from build123d import *

# Parameters (mm, degrees)
SKETCH1_R           = 150
SKETCH1_W           = 33
SKETCH1_H           = 33
BOSS_EXTRUDE1_DEPTH = 5
SKETCH4_R           = 1.5
CUT_EXTRUDE1_DEPTH  = 55
CIRPATTERN1_COUNT   = 12
CUT_EXTRUDE2_REACH  = 214.368
SKETCH5_W           = 20
SKETCH5_H           = 5
SKETCH5_W_2         = 5
SKETCH5_H_2         = 20
CUT_EXTRUDE3_DEPTH  = 10
BOSS_EXTRUDE2_DEPTH = 5
CUT_EXTRUDE4_DEPTH  = 5
BOSS_EXTRUDE3_DEPTH = 15
SKETCH11_W          = 22.5
SKETCH11_H          = 8
BOSS_EXTRUDE4_DEPTH = 3


with BuildPart() as part:
    # Sketch1 → Boss-Extrude1 (new, symmetric)
    with BuildSketch(Plane.XY):
        Circle(SKETCH1_R)
        Polygon((37.460580838, 97.883629292), (66.039419162, 81.383629292), (82.539419162, 109.962467617), (53.960580838, 126.462467617), align=None, mode=Mode.SUBTRACT)
        with Locations((0, 120)):
            Rectangle(SKETCH1_W, SKETCH1_H, mode=Mode.SUBTRACT)
        Polygon((81.383629292, 66.039419162), (97.883629292, 37.460580838), (126.462467617, 53.960580838), (109.962467617, 82.539419162), align=None, mode=Mode.SUBTRACT)
        with Locations((120, 0)):
            Rectangle(SKETCH1_W, SKETCH1_H, mode=Mode.SUBTRACT)
        Polygon((97.883629292, -37.460580838), (81.383629292, -66.039419162), (109.962467617, -82.539419162), (126.462467617, -53.960580838), align=None, mode=Mode.SUBTRACT)
        Polygon((66.039419162, -81.383629292), (37.460580838, -97.883629292), (53.960580838, -126.462467617), (82.539419162, -109.962467617), align=None, mode=Mode.SUBTRACT)
        with Locations((0, -120)):
            Rectangle(SKETCH1_W, SKETCH1_H, mode=Mode.SUBTRACT)
        Polygon((-37.460580838, -97.883629292), (-66.039419162, -81.383629292), (-82.539419162, -109.962467617), (-53.960580838, -126.462467617), align=None, mode=Mode.SUBTRACT)
        Polygon((-81.383629292, -66.039419162), (-97.883629292, -37.460580838), (-126.462467617, -53.960580838), (-109.962467617, -82.539419162), align=None, mode=Mode.SUBTRACT)
        with Locations((-120, 0)):
            Rectangle(SKETCH1_W, SKETCH1_H, mode=Mode.SUBTRACT)
        Polygon((-97.883629292, 37.460580838), (-81.383629292, 66.039419162), (-109.962467617, 82.539419162), (-126.462467617, 53.960580838), align=None, mode=Mode.SUBTRACT)
        Polygon((-66.039419162, 81.383629292), (-37.460580838, 97.883629292), (-53.960580838, 126.462467617), (-82.539419162, 109.962467617), align=None, mode=Mode.SUBTRACT)
    extrude(amount=BOSS_EXTRUDE1_DEPTH, both=True)

    # Sketch4 → Cut-Extrude1 (cut)
    with BuildSketch(Plane(origin=(0, -150, 0), x_dir=(-1, 0, 0), z_dir=(0, -1, 0))):
        with Locations(Location((0, 0, 0), (0, 0, 90))):
            Circle(SKETCH4_R)
    cut_extrude1 = extrude(amount=-CUT_EXTRUDE1_DEPTH, mode=Mode.SUBTRACT)

    # CirPattern1: Cut-Extrude1 ×12 about axis
    cirpattern1_axis = Axis((0, 0, 0), (0, 0, 1))
    for i in range(1, CIRPATTERN1_COUNT):
        add(cut_extrude1.rotate(cirpattern1_axis, i * 360 / CIRPATTERN1_COUNT), mode=Mode.SUBTRACT)

    # Sketch5 → Cut-Extrude2 (cut, up to next)
    with BuildSketch(Plane(origin=(0, 0, -5), x_dir=(-1, 0, 0), z_dir=(0, 0, -1)), mode=Mode.PRIVATE) as cut_extrude2_sk1:
        Polygon((38.089745962, 85.973375254), (55.410254038, 75.973375254), (57.910254038, 80.303502273), (40.589745962, 90.303502273), align=None)
    cut_extrude2_tool1 = extrude(cut_extrude2_sk1.sketch, amount=-CUT_EXTRUDE2_REACH, mode=Mode.PRIVATE) & part.part
    # Sketch5 → Cut-Extrude2 (cut, up to next)
    with BuildSketch(Plane(origin=(0, 0, -5), x_dir=(-1, 0, 0), z_dir=(0, 0, -1)), mode=Mode.PRIVATE) as cut_extrude2_sk2:
        with Locations((0, 96)):
            Rectangle(SKETCH5_W, SKETCH5_H)
    cut_extrude2_tool2 = extrude(cut_extrude2_sk2.sketch, amount=-CUT_EXTRUDE2_REACH, mode=Mode.PRIVATE) & part.part
    # Sketch5 → Cut-Extrude2 (cut, up to next)
    with BuildSketch(Plane(origin=(0, 0, -5), x_dir=(-1, 0, 0), z_dir=(0, 0, -1)), mode=Mode.PRIVATE) as cut_extrude2_sk3:
        Polygon((75.973375254, 55.410254038), (85.973375254, 38.089745962), (90.303502273, 40.589745962), (80.303502273, 57.910254038), align=None)
    cut_extrude2_tool3 = extrude(cut_extrude2_sk3.sketch, amount=-CUT_EXTRUDE2_REACH, mode=Mode.PRIVATE) & part.part
    # Sketch5 → Cut-Extrude2 (cut, up to next)
    with BuildSketch(Plane(origin=(0, 0, -5), x_dir=(-1, 0, 0), z_dir=(0, 0, -1)), mode=Mode.PRIVATE) as cut_extrude2_sk4:
        with Locations((96, 0)):
            Rectangle(SKETCH5_W_2, SKETCH5_H_2)
    cut_extrude2_tool4 = extrude(cut_extrude2_sk4.sketch, amount=-CUT_EXTRUDE2_REACH, mode=Mode.PRIVATE) & part.part
    # Sketch5 → Cut-Extrude2 (cut, up to next)
    with BuildSketch(Plane(origin=(0, 0, -5), x_dir=(-1, 0, 0), z_dir=(0, 0, -1)), mode=Mode.PRIVATE) as cut_extrude2_sk5:
        Polygon((85.973375254, -38.089745962), (75.973375254, -55.410254038), (80.303502273, -57.910254038), (90.303502273, -40.589745962), align=None)
    cut_extrude2_tool5 = extrude(cut_extrude2_sk5.sketch, amount=-CUT_EXTRUDE2_REACH, mode=Mode.PRIVATE) & part.part
    # Sketch5 → Cut-Extrude2 (cut, up to next)
    with BuildSketch(Plane(origin=(0, 0, -5), x_dir=(-1, 0, 0), z_dir=(0, 0, -1)), mode=Mode.PRIVATE) as cut_extrude2_sk6:
        Polygon((55.410254038, -75.973375254), (38.089745962, -85.973375254), (40.589745962, -90.303502273), (57.910254038, -80.303502273), align=None)
    cut_extrude2_tool6 = extrude(cut_extrude2_sk6.sketch, amount=-CUT_EXTRUDE2_REACH, mode=Mode.PRIVATE) & part.part
    # Sketch5 → Cut-Extrude2 (cut, up to next)
    with BuildSketch(Plane(origin=(0, 0, -5), x_dir=(-1, 0, 0), z_dir=(0, 0, -1)), mode=Mode.PRIVATE) as cut_extrude2_sk7:
        with Locations((0, -96)):
            Rectangle(SKETCH5_W, SKETCH5_H)
    cut_extrude2_tool7 = extrude(cut_extrude2_sk7.sketch, amount=-CUT_EXTRUDE2_REACH, mode=Mode.PRIVATE) & part.part
    # Sketch5 → Cut-Extrude2 (cut, up to next)
    with BuildSketch(Plane(origin=(0, 0, -5), x_dir=(-1, 0, 0), z_dir=(0, 0, -1)), mode=Mode.PRIVATE) as cut_extrude2_sk8:
        Polygon((-38.089745962, -85.973375254), (-55.410254038, -75.973375254), (-57.910254038, -80.303502273), (-40.589745962, -90.303502273), align=None)
    cut_extrude2_tool8 = extrude(cut_extrude2_sk8.sketch, amount=-CUT_EXTRUDE2_REACH, mode=Mode.PRIVATE) & part.part
    # Sketch5 → Cut-Extrude2 (cut, up to next)
    with BuildSketch(Plane(origin=(0, 0, -5), x_dir=(-1, 0, 0), z_dir=(0, 0, -1)), mode=Mode.PRIVATE) as cut_extrude2_sk9:
        Polygon((-75.973375254, -55.410254038), (-85.973375254, -38.089745962), (-90.303502273, -40.589745962), (-80.303502273, -57.910254038), align=None)
    cut_extrude2_tool9 = extrude(cut_extrude2_sk9.sketch, amount=-CUT_EXTRUDE2_REACH, mode=Mode.PRIVATE) & part.part
    # Sketch5 → Cut-Extrude2 (cut, up to next)
    with BuildSketch(Plane(origin=(0, 0, -5), x_dir=(-1, 0, 0), z_dir=(0, 0, -1)), mode=Mode.PRIVATE) as cut_extrude2_sk10:
        with Locations((-96, 0)):
            Rectangle(SKETCH5_W_2, SKETCH5_H_2)
    cut_extrude2_tool10 = extrude(cut_extrude2_sk10.sketch, amount=-CUT_EXTRUDE2_REACH, mode=Mode.PRIVATE) & part.part
    # Sketch5 → Cut-Extrude2 (cut, up to next)
    with BuildSketch(Plane(origin=(0, 0, -5), x_dir=(-1, 0, 0), z_dir=(0, 0, -1)), mode=Mode.PRIVATE) as cut_extrude2_sk11:
        Polygon((-85.973375254, 38.089745962), (-75.973375254, 55.410254038), (-80.303502273, 57.910254038), (-90.303502273, 40.589745962), align=None)
    cut_extrude2_tool11 = extrude(cut_extrude2_sk11.sketch, amount=-CUT_EXTRUDE2_REACH, mode=Mode.PRIVATE) & part.part
    # Sketch5 → Cut-Extrude2 (cut, up to next)
    with BuildSketch(Plane(origin=(0, 0, -5), x_dir=(-1, 0, 0), z_dir=(0, 0, -1)), mode=Mode.PRIVATE) as cut_extrude2_sk12:
        Polygon((-55.410254038, 75.973375254), (-38.089745962, 85.973375254), (-40.589745962, 90.303502273), (-57.910254038, 80.303502273), align=None)
    cut_extrude2_tool12 = extrude(cut_extrude2_sk12.sketch, amount=-CUT_EXTRUDE2_REACH, mode=Mode.PRIVATE) & part.part
    add(cut_extrude2_tool1.solids().sort_by_distance((-48, 83.138439, -5))[0], mode=Mode.SUBTRACT)
    add(cut_extrude2_tool2.solids().sort_by_distance((0, 96, -5))[0], mode=Mode.SUBTRACT)
    add(cut_extrude2_tool3.solids().sort_by_distance((-83.138439, 48, -5))[0], mode=Mode.SUBTRACT)
    add(cut_extrude2_tool4.solids().sort_by_distance((-96, 0, -5))[0], mode=Mode.SUBTRACT)
    add(cut_extrude2_tool5.solids().sort_by_distance((-83.138439, -48, -5))[0], mode=Mode.SUBTRACT)
    add(cut_extrude2_tool6.solids().sort_by_distance((-48, -83.138439, -5))[0], mode=Mode.SUBTRACT)
    add(cut_extrude2_tool7.solids().sort_by_distance((0, -96, -5))[0], mode=Mode.SUBTRACT)
    add(cut_extrude2_tool8.solids().sort_by_distance((48, -83.138439, -5))[0], mode=Mode.SUBTRACT)
    add(cut_extrude2_tool9.solids().sort_by_distance((83.138439, -48, -5))[0], mode=Mode.SUBTRACT)
    add(cut_extrude2_tool10.solids().sort_by_distance((96, 0, -5))[0], mode=Mode.SUBTRACT)
    add(cut_extrude2_tool11.solids().sort_by_distance((83.138439, 48, -5))[0], mode=Mode.SUBTRACT)
    add(cut_extrude2_tool12.solids().sort_by_distance((48, 83.138439, -5))[0], mode=Mode.SUBTRACT)

    # Sketch6 → Cut-Extrude3 (cut)
    with BuildSketch(Plane.XY.offset(5)):
        with BuildLine():
            Line((1.811733316, 6.761480784), (0, 0))
            Line((0, 0), (-1.811733316, 6.761480784))
            Line((-1.811733316, 6.761480784), (-38.822856765, 144.888873943))
            ThreePointArc((-38.822856765, 144.888873943), (-91.314214351, -119.003001044), (150, 0))
            ThreePointArc((150, 0), (119.003001044, 91.314214351), (38.822856765, 144.888873943))
            Line((38.822856765, 144.888873943), (1.811733316, 6.761480784))
        make_face()
        with BuildLine():
            Line((-1.811733316, 6.761480784), (0, 0))
            Line((0, 0), (1.811733316, 6.761480784))
            ThreePointArc((1.811733316, 6.761480784), (0, 7), (-1.811733316, 6.761480784))
        make_face()
    extrude(amount=-CUT_EXTRUDE3_DEPTH, mode=Mode.SUBTRACT)

    # Sketch7 → Boss-Extrude2 (add)
    with BuildSketch(Plane.XY.offset(5)):
        Polygon((-20.358771838, 56.661454352), (-15.529142706, 57.955549577), (-16.823237932, 62.785178709), (-21.652867063, 61.491083483), (-22.946962289, 66.320712615), (-27.77659142, 65.026617389), (-23.894305744, 50.537729995), (-19.064676612, 51.83182522), align=None)
        Polygon((-37.182009769, 119.446633061), (-32.352380638, 120.740728286), (-33.646475863, 125.570357418), (-38.476104995, 124.276262192), (-39.77020022, 129.105891324), (-44.599829352, 127.811796098), (-40.717543675, 113.322908704), (-35.887914544, 114.617003929), align=None)
    extrude(amount=-BOSS_EXTRUDE2_DEPTH)

    # Sketch9 → Cut-Extrude4 (cut)
    with BuildSketch(Plane.XY.offset(5)):
        Polygon((15.529142706, 57.955549577), (16.823237932, 62.785178709), (11.9936088, 64.079273934), (13.287704026, 68.908903066), (8.458074894, 70.202998291), (4.575789218, 55.714110897), (9.405418349, 54.420015671), (10.699513575, 59.249644803), align=None)
        Polygon((32.352380638, 120.740728286), (33.646475863, 125.570357418), (28.816846732, 126.864452643), (30.110941957, 131.694081775), (25.281312826, 132.988177), (21.399027149, 118.499289606), (26.228656281, 117.20519438), (27.522751506, 122.034823512), align=None)
    extrude(amount=-CUT_EXTRUDE4_DEPTH, mode=Mode.SUBTRACT)

    # Sketch10 → Boss-Extrude3 (add)
    with BuildSketch(Plane.XY.offset(5)):
        Polygon((-7, 82.5), (-10, 82.5), (-12.143593539, 74.5), (-10, 74.5), (-7, 74.5), align=None)
        Polygon((22.105808376, 82.5), (15.5, 82.5), (15.5, 74.5), (19.962214836, 74.5), align=None)
    extrude(amount=BOSS_EXTRUDE3_DEPTH)

    # Sketch11 → Boss-Extrude4 (add)
    with BuildSketch(Plane.XY.offset(5)):
        with Locations((4.25, 78.5)):
            Rectangle(SKETCH11_W, SKETCH11_H)
    extrude(amount=BOSS_EXTRUDE4_DEPTH)


solid = part.part
Design review of the part built by this model. Coordinates are the model's own, in mm. A direction names the side the tool comes from. Give positions to 0.01 mm unless a question says otherwise; leave off trailing zeros. Order: outer loops, then holes, each group sorted by start corner. A loop starts at its lowest first (then second) coordinate and runs counter-clockwise, first axis right, second up.
1. Mouldability with a two-part tool opening along Z and no side actions: class faces 1 (the flat face through (11, 62, 0)), 2 (the flat face through (6.957, 55.076, 2.535)), 3 (the cylindrical face through (-0.45, 143.34, -1.43)) as +Z half, -Z half, draft (parallel to the pull), parting line (faces both ways), or undercut.
Solution:
face 1: +Z half
face 2: draft
face 3: undercut
2. For pin 1 Ø6 at (x, y) = (-22, 59) entering from -Z; pin 2 Ø6 at (x, y) = (11, 63.5) entering from +Z; pin 3 Ø1.5 at (y, z) = (97, 0.5) entering from -X; pin 4 Ø10 at (y, z) = (59, 13.5) entering from +X, all flat-tipped, find the tip position at first contact; note any pin that passes through.
Solution:
pin 1: stops at z = 0
pin 2: stops at z = 5
pin 3: stops at x = -26.19
pin 4: passes through
3. Tool access review of faces 4 (the flat face through (27.73, 132.33, 2.54)), 5 (the flat face through (16.5, 120, 0)), 6 (the flat face through (-22, 59, 0)): name each direction out of +Z, -Z, +X, -X, +Y, -Y from which nothing blocks a thin tool from reaching the whole face with its end or side.
Solution:
face 4: +Z
face 5: +Z, -Z
face 6: -Z, -X, -Y
4. Add section B-B, the plane x = 0. State the section outline as (y, z) points, then the cut area to 3 significant figures.
Solution:
outline: (7, -5) - (93.5, -5) - (93.5, 5) - (82.5, 5) - (82.5, 8) - (74.5, 8) - (74.5, 5) - (7, 5) - close; (98.5, -5) - (103.5, -5) - (103.5, -1.5) - (98.5, -1.5) - close; (98.5, 1.5) - (103.5, 1.5) - (103.5, 5) - (98.5, 5) - close; (136.5, -5) - (150, -5) - (150, -1.5) - (136.5, -1.5) - close; (136.5, 1.5) - (150, 1.5) - (150, 5) - (136.5, 5) - close
area: 1,020 mm2
5. Add section C-C, the plane y = 79.5. State the section outline as (x, z) points.
Solution:
outline: (-21.3, -5) - (21.3, -5) - (21.3, 20) - (15.5, 20) - (15.5, 8) - (-7, 8) - (-7, 20) - (-10.8, 20) - (-10.8, 5) - (-21.3, 5) - close
6. Add section D-D, the plane y = 30.5. State the section outline as (x, z) points, then the cut area to 3 significant figures.
Solution:
outline: (-8.17, -5) - (8.17, -5) - (8.17, 5) - (-8.17, 5) - close
area: 163 mm2
7. To check wall thickness, follow L1, parallel to Z at x = -9, y = 40.5; L2, parallel to Y at x = 17, z = 9.25; L3, parallel to X at y = 142.75, z = 0. State the ranges of each line that lie inside material, in increasing order.
Solution:
L1: z = -5 to 5
L2: y = 74.5 to 82.5
L3: x = -38.25 to -1.5, 1.5 to 38.25
8. Add section A-A, the plane z = 13. State the section outline as (x, y) points, then the cut area to 3 significant figures.
Solution:
outline: (-12.14, 74.5) - (-7, 74.5) - (-7, 82.5) - (-10, 82.5) - close; (15.5, 74.5) - (19.96, 74.5) - (22.11, 82.5) - (15.5, 82.5) - close
area: 76.8 mm2
